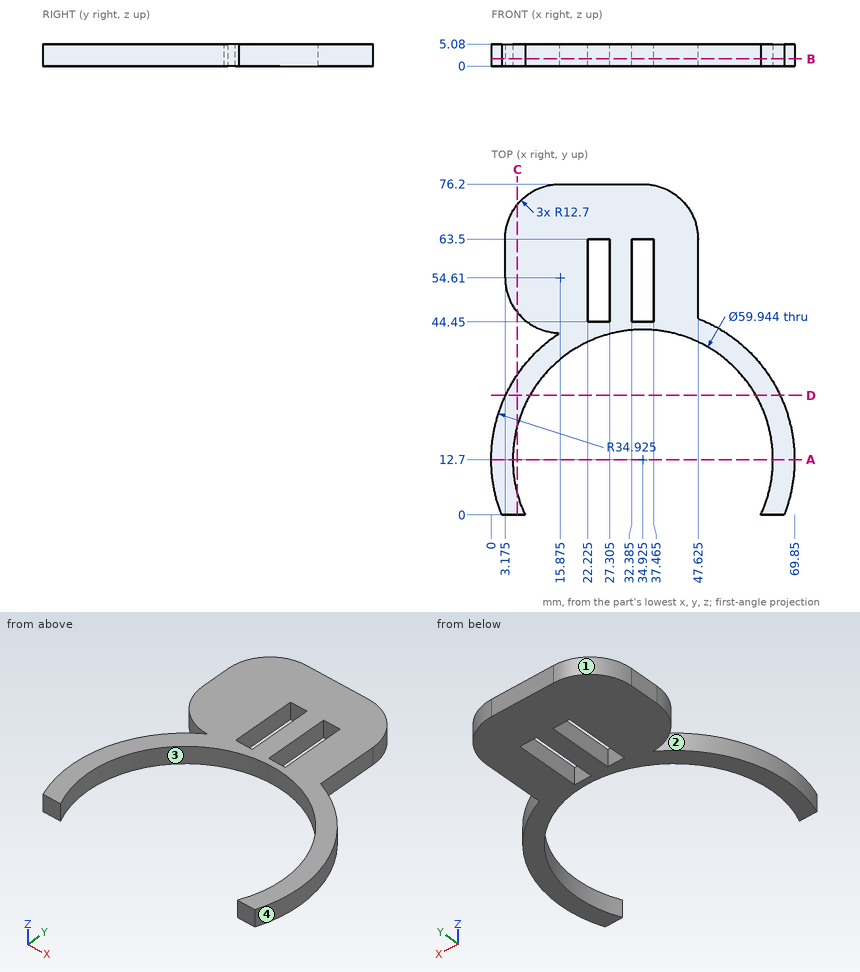
Geometry: see drawing. Coordinates: mm, zero at the bounding-box minimum. Give positions to 0.01 mm unless a question says otherwise; leave off trailing zeros. Order: outer loops, then holes, each group sorted by start corner. A loop starts at its lowest first (then second) coordinate and runs counter-clockwise, first axis right, second up.
1. Pin query (flat end, axial travel): pin 1 Ø2.5 at (x, z) = (34.5, 2) entering from -Y; pin 2 Ø3 at (x, y) = (35, 41) entering from +Z; pin 3 Ø1.5 at (y, z) = (53, 3.5) entering from +X (3 decimals); pin 4 Ø1 at (x, z) = (43, 1) entering from -Y. Return the tip coordinate at first contact, or that it passes through.
Computed:
pin 1: stops at y = 42.63
pin 2: passes through
pin 3: stops at x = 47.625
pin 4: stops at y = 41.42
2. Cut plane A-A (y = 12.7). Return loops of the section in (x, z).
Computed:
outline: (0, 0) - (4.95, 0) - (4.95, 5.08) - (0, 5.08) - close; (64.9, 0) - (69.85, 0) - (69.85, 5.08) - (64.9, 5.08) - close
3. Cut plane B-B (z = 1.65). Return loops of the section in (x, y) (3 decimals), and give its area (3 significant figures).
Computed:
outline: (2.391, 0) - (7.777, 0) arc R29.972 cw (long way) to (62.073, 0) - (67.459, 0) arc R34.925 ccw to (47.625, 45.234) - (47.625, 63.5) arc R12.7 ccw to (34.925, 76.2) - (15.875, 76.2) arc R12.7 ccw to (3.175, 63.5) - (3.175, 54.61) arc R12.7 ccw to (15.781, 41.91) arc R34.925 ccw to start; hole (22.225, 44.45) - (27.305, 44.45) - (27.305, 63.5) - (22.225, 63.5) - close; hole (32.385, 44.45) - (37.465, 44.45) - (37.465, 63.5) - (32.385, 63.5) - close
area: 1,720 mm2
4. Cut plane C-C (x = 6). Return loops of the section in (y, z), and give its area (3 significant figures).
Computed:
outline: (0, 0) - (4.85, 0) - (4.85, 5.08) - (0, 5.08) - close; (20.55, 0) - (32.27, 0) - (32.27, 5.08) - (20.55, 5.08) - close; (46.62, 0) - (71.49, 0) - (71.49, 5.08) - (46.62, 5.08) - close
area: 210 mm2
5. Cut plane D-D (y = 27.5). Return loops of the section in (x, z), and give its area (3 significant figures).
Computed:
outline: (3.29, 0) - (8.86, 0) - (8.86, 5.08) - (3.29, 5.08) - close; (60.99, 0) - (66.56, 0) - (66.56, 5.08) - (60.99, 5.08) - close
area: 56.6 mm2
6. Line query: probe 1 along X at (y, z) = (60, 2.9) (3 decimals); probe 2 along X at (y, z) = (12.7, 2.6); probe 3 along Y at (x, z) = (11.5, 2.35). Output: solid intervals per line, ascending.
Computed:
probe 1: x = 3.175 to 22.225, 27.305 to 32.385, 37.465 to 47.625
probe 2: x = 0 to 4.95, 64.9 to 69.85
probe 3: y = 31.4 to 38.6, 42.69 to 75.42
7. Draft query along Y for the marked faces 1, 2, 3 and 4. Return one class per face: released by +Y, released by -Y, zero draft, split by the parting line, or undercut.
Computed:
face 1: released by +Y
face 2: undercut
face 3: undercut
face 4: split by the parting line
